Input: part model. Units: mm. Frame: model coordinates. Give positions to 0.01 mm unless a question says otherwise; leave off trailing zeros. Loops run counter-clockwise (first coordinate to the right, second up) from the corner with the lowest first, then second, coordinate; pieces in that order, holes last. Notation, with made-up numbers: M 77,-21 L 136,-21 A25 cw 136,0 Z; hole C -32,79 d6. An arc over 180 degrees is marked long. Answer as a JSON object with one key per item and string values. Group by question number.
1) Draft query along X for faces 1 (the cylindrical face through (4.024, -6.833, -0.601)), 2 (the cylindrical face through (-1.08, -4.88, -4.14)), 3 (the flat face through (-4.191, 7.396, -5.155)), 4 (the flat face through (-5, 2, 0)). Return one class per face: +X half, -X half, draft (parallel to the pull), parting line (faces both ways), or undercut.
2) Section query A-A on y = 0. Return loops of the section in (x, z).
3) Section query C-C on z = -1. Return loops of the section in (x, y), plus the area to 3 significant figures.
4) Ray query, L1, parallel to X at y = -4, z = -1.5; L2, parallel to Y at x = -2.5, z = -6; L3, parallel to Y at x = 1.5, z = -3. Return the intervals inside material, ascending.
5) First-contact query: P1, Ø1, axis at x = -5, z = -3, coming from the +Y side; P2, Ø3, axis at x = -5, z = -3.5, coming from the +Y side. Flat tips, straight axial feed; report the tip coordinate or a pass-through.
6) Section query B-B on z = -6. Return loops of the section in (x, y).
from build123d import *

# Parameters (mm, degrees)
ESQUISSE1_R        = 5
BOSS_EXTRU_1_DEPTH = 8.4
CONG_2_R           = 2


with BuildPart() as part:
    # Esquisse1 → Boss.-Extru.1 (new body)
    with BuildSketch(Plane.XY):
        Polygon((8.5, 4.907477288), (0, 9.814954576), (-8.5, 4.907477288), (-8.5, -4.907477288), (0, -9.814954576), (8.5, -4.907477288), align=None)
        Circle(ESQUISSE1_R, mode=Mode.SUBTRACT)
    extrude(amount=-BOSS_EXTRU_1_DEPTH)

    # Congé2
    cong_2_edges = [part.edges().sort_by_distance(p)[0] for p in [
        (4.25, -7.361215932, 0),
        (-4.25, -7.361215932, 0),
        (-8.5, 0, 0),
        (-4.25, 7.361215932, 0),
        (4.25, 7.361215932, 0),
        (8.5, 0, 0),
    ]]
    fillet(cong_2_edges, radius=CONG_2_R)


solid = part.part
Output:
{
 "1": {"face 1": "+X half", "face 2": "undercut", "face 3": "-X half", "face 4": "draft"},
 "2": {"outline": "M -8.5,-8.4 L -5,-8.4 L -5,0 L -6.5,0 A2 ccw -8.5,-2 Z; M 5,-8.4 L 8.5,-8.4 L 8.5,-2 A2 ccw 6.5,0 L 5,0 Z"},
 "3": {"outline": "M -8.23,-4.75 L 0,-9.51 L 8.23,-4.75 L 8.23,4.75 L 0,9.51 L -8.23,4.75 Z; hole C 0,0 d10", "area": "156 mm^2"},
 "4": {"L1": "x = -8.44 to -3, 3 to 8.44", "L2": "y = -8.37 to -4.33, 4.33 to 8.37", "L3": "y = -8.95 to -4.77, 4.77 to 8.95"},
 "5": {"P1": "stops at y = 7.22", "P2": "stops at y = 7.79"},
 "6": {"outline": "M -8.5,-4.91 L 0,-9.81 L 8.5,-4.91 L 8.5,4.91 L 0,9.81 L -8.5,4.91 Z; hole C 0,0 d10"}
}
